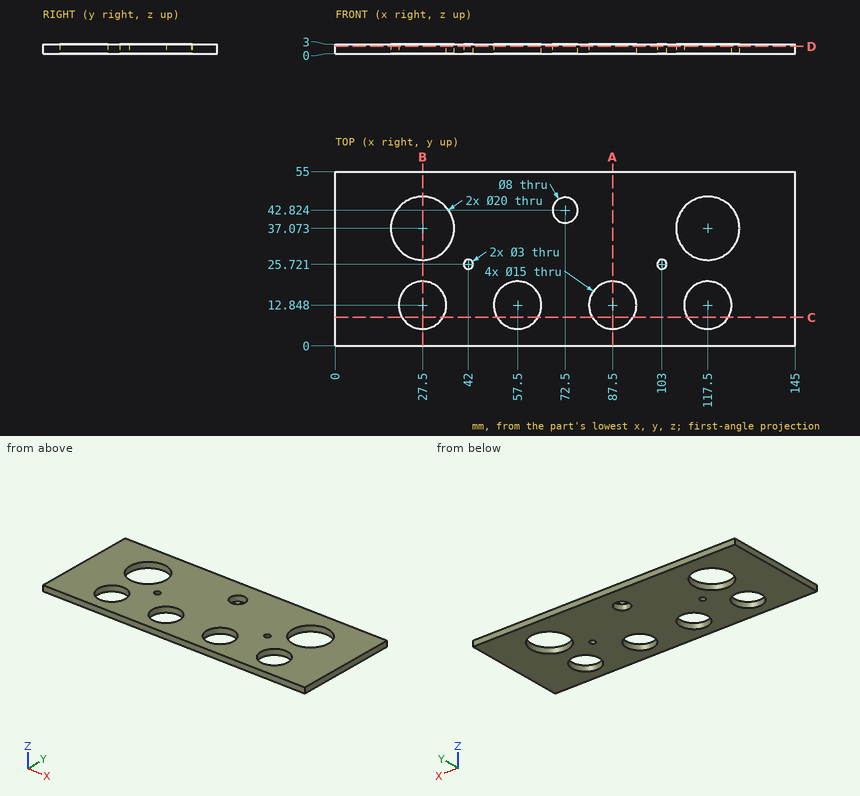
Source: three-view drawing plus pictorial views. Frame: mm from the lowest corner of the part. Round coordinates to 2 decimals unless told otherwise and drop trailing zeros. Loops run counter-clockwise (first coordinate to the right, second up) from the corner with the lowest first, then second, coordinate; pieces in that order, holes last.
Q1. Section D-D, the plane z = 2.25. State how many separate pieces and enclosed holes the cut face has.
Q2. Section A-A, the plane x = 87.5. Return loops of the section in (y, z), plus the area to 3 significant figures.
Q3. Section B-B, the plane x = 27.5. Return loops of the section in (y, z).
Q4. Ray query, line 1 (X direction, y = 12.5, z = 1.25); line 2 (X direction, y = 25.5, z = 0.4); line 3 (X direction, y = 39.5, z = 2.05) (1 decimal). Return the intervals inside material, ascending.
Q5. Section C-C, the plane y = 9. Return loops of the section in (x, z).
Q6. First-contact query: P1, Ø18, axis at x = 27.5, y = 37.07, coming from the +Z side. Flat tip, straight axial feed; report the tip coordinate or a pass-through.
Solutions:
1. separate pieces: 1
1. enclosed holes: 9
2. outline: (0, 0) - (5.35, 0) - (5.35, 3) - (0, 3) - close; (20.35, 0) - (55, 0) - (55, 3) - (20.35, 3) - close
2. area: 120 mm2
3. outline: (0, 0) - (5.35, 0) - (5.35, 3) - (0, 3) - close; (20.35, 0) - (27.07, 0) - (27.07, 3) - (20.35, 3) - close; (47.07, 0) - (55, 0) - (55, 3) - (47.07, 3) - close
4. line 1: x = 0 to 20.01, 34.99 to 50.01, 64.99 to 80.01, 94.99 to 110.01, 124.99 to 145
4. line 2: x = 0 to 40.52, 43.48 to 101.52, 104.48 to 145
4. line 3: x = 0 to 17.8, 37.2 to 70.3, 74.7 to 107.8, 127.2 to 145
5. outline: (0, 0) - (21.06, 0) - (21.06, 3) - (0, 3) - close; (33.94, 0) - (51.06, 0) - (51.06, 3) - (33.94, 3) - close; (63.94, 0) - (81.06, 0) - (81.06, 3) - (63.94, 3) - close; (93.94, 0) - (111.06, 0) - (111.06, 3) - (93.94, 3) - close; (123.94, 0) - (145, 0) - (145, 3) - (123.94, 3) - close
6. P1: passes through
